Input: dimensioned drawing with shaded views. Units: mm. Origin: part minimum x, y, z. Give positions to 0.01 mm unless a question says otherwise; leave off trailing zeros. Write each loop counter-clockwise with the first axis right and the second up, starting at its lowest first coordinate (ties: lowest second). Pieces come first, ordered by that corner, then holes. Notation, with made-up numbers: (25.25, 87) -> (70.25, 87) arc R20 ccw to (70.25, 115) -> close; hole circle Ø11 at (-14.75, -4). An arc over 180 degrees is marked (long way). Answer as a JSON object with one key per item and string values.
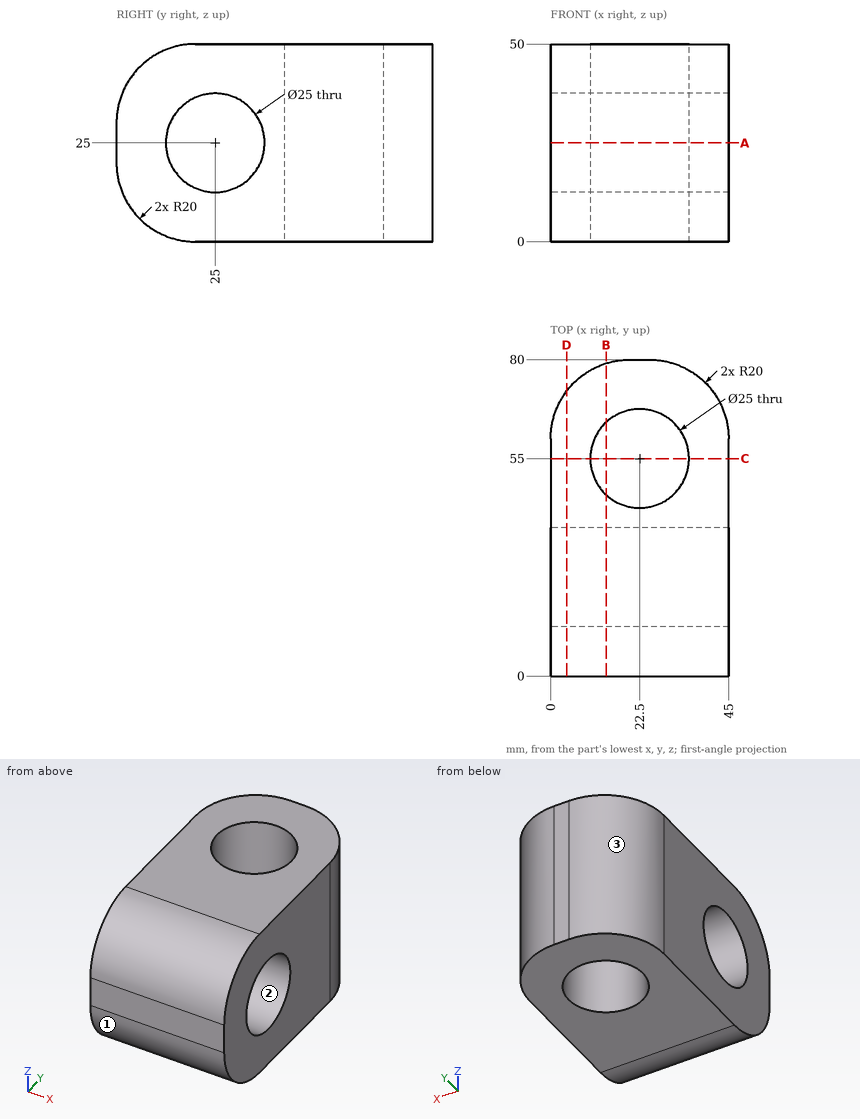
Q1. Cut plane D-D (x = 4). Return the cut outline in (y, z).
Values:
{"outline": "(0, 20) arc R20 ccw to (20, 0) -> (72, 0) -> (72, 50) -> (20, 50) arc R20 ccw to (0, 30) -> close; hole circle Ø25 at (25, 25)"}
Q2. Mould query, pull axis Y, two halves, no side actions, for the marked faces 1, 2 and 3. Classes: pulls with the +Y half, pulls with the -Y half, needs draft (parallel to the pull), parting line crosses it, or undercut.
Values:
{"face 1": "pulls with the -Y half", "face 2": "undercut", "face 3": "pulls with the +Y half"}
Q3. Cut plane A-A (z = 25). Return the cut outline in (x, y).
Values:
{"outline": "(0, 0) -> (45, 0) -> (45, 12.5) -> (0, 12.5) -> close; (0, 37.5) -> (45, 37.5) -> (45, 60) arc R20 ccw to (25, 80) -> (20, 80) arc R20 ccw to (0, 60) -> close; hole circle Ø25 at (22.5, 55)"}
Q4. Cut plane C-C (y = 55). Return the cut outline in (x, z).
Values:
{"outline": "(0, 0) -> (10, 0) -> (10, 50) -> (0, 50) -> close; (35, 0) -> (45, 0) -> (45, 50) -> (35, 50) -> close"}
Q5. First-contact query: P1, Ø8, axis at x = 21, z = 42.5, coming from the -Y side; P2, Ø2, axis at x = 13.5, z = 14.5, coming from the +Y side; P3, Ø20, axis at x = 22.5, y = 55, coming from the -Z side; P4, Ø1.5, axis at x = 39.5, z = 24.5, coming from the +Y side. Flat tips, straight axial feed; report the tip coordinate or a pass-through.
Values:
{"P1": "y = 1.9", "P2": "y = 79.23", "P3": "through", "P4": "y = 74.52"}
Q6. Material intervals for L1, parallel to Y at x = 16, z = 15; L2, parallel to Y at x = 26, z = 25; L3, parallel to Z at x = 11, y = 31, sorted ascending. Write a range as from..to.
Values:
{"L1": "0.64..17.5, 32.5..44.32, 65.68..79.6", "L2": "0..12.5, 37.5..43, 67..79.97", "L3": "0..14.03, 35.97..50"}
Q7. Cut plane B-B (x = 14). Return the cut outline in (y, z).
Values:
{"outline": "(0, 20) arc R20 ccw to (20, 0) -> (45.83, 0) -> (45.83, 50) -> (20, 50) arc R20 ccw to (0, 30) -> close; (64.17, 0) -> (79.08, 0) -> (79.08, 50) -> (64.17, 50) -> close; hole circle Ø25 at (25, 25)"}
